from build123d import *

# Parameters (mm, degrees)
BOSS_EXTRUDE1_DEPTH = 30.3
SKETCH2_R           = 2.5527
CUT_EXTRUDE1_DEPTH  = 62.816745304
CUT_EXTRUDE2_DEPTH  = 62.816745304


with BuildPart() as part:
    # Sketch1 → Boss-Extrude1 (new body)
    with BuildSketch(Plane(origin=(0, 0, 0), x_dir=(1, 0, 0), z_dir=(0, 1, 0))):
        Polygon((0, 0), (38.1, 0), (38.1, -18), (18, -18), (18, -38.1), (0, -38.1), align=None)
    extrude(amount=BOSS_EXTRUDE1_DEPTH)

    # Sketch2 → Cut-Extrude1 (cut, through all)
    with BuildSketch(Plane(origin=(0, 30.3, 0), x_dir=(1, 0, 0), z_dir=(0, 1, 0))):
        with Locations(Location((6.35, -6.35, 0), (0, 0, 270))):
            Circle(SKETCH2_R)
        with Locations(Location((19.05, -6.35, 0), (0, 0, 270))):
            Circle(SKETCH2_R)
        with Locations(Location((31.75, -6.35, 0), (0, 0, 270))):
            Circle(SKETCH2_R)
        with Locations(Location((6.35, -19.05, 0), (0, 0, 270))):
            Circle(SKETCH2_R)
        with Locations(Location((6.35, -31.75, 0), (0, 0, 270))):
            Circle(SKETCH2_R)
    extrude(amount=-CUT_EXTRUDE1_DEPTH, mode=Mode.SUBTRACT)

    # Sketch3 → Cut-Extrude2 (cut, through all)
    with BuildSketch(Plane(origin=(0, 30.3, 0), x_dir=(1, 0, 0), z_dir=(0, 1, 0))):
        with BuildLine():
            Line((0, -6.35), (-3.023343313, -6.35))
            Line((-3.023343313, -6.35), (-3.023343313, 2.931868043))
            Line((-3.023343313, 2.931868043), (6.35, 2.931868043))
            Line((6.35, 2.931868043), (6.35, 0))
            ThreePointArc((6.35, 0), (1.859871939, -1.859871939), (0, -6.35))
        make_face()
    extrude(amount=-CUT_EXTRUDE2_DEPTH, mode=Mode.SUBTRACT)


solid = part.part
The listing builds one solid part. Answer for the finished solid, in the listing's coordinates (mm). A direction names the side the tool comes from. Give positions to 0.01 mm unless a question says otherwise; leave off trailing zeros. Loops run counter-clockwise (first coordinate to the right, second up) from the corner with the lowest first, then second, coordinate; pieces in that order, holes last. Notation, with made-up numbers: (-18.5, -21.75) - (-13.5, -21.75) arc R26 cw to (-13.5, 17.25) - close; hole circle Ø8 at (-35.75, -28.5). An arc over 180 degrees is marked (long way). Write each question's results on one line, items separated by ' | '.
1. Find section D-D, the plane x = 5. Write down the section's boundary in (y, z), then the cut area to 3 significant figures.
Resolved:
outline: (0, 0.15) - (30.3, 0.15) - (30.3, 4.18) - (0, 4.18) - close; (0, 8.52) - (30.3, 8.52) - (30.3, 16.88) - (0, 16.88) - close; (0, 21.22) - (30.3, 21.22) - (30.3, 29.58) - (0, 29.58) - close; (0, 33.92) - (30.3, 33.92) - (30.3, 38.1) - (0, 38.1) - close | area: 756 mm^2
2. Find section C-C, the plane x = 31.75. Write down the section's boundary in (y, z), then the cut area to 3 significant figures.
Resolved:
outline: (0, 0) - (30.3, 0) - (30.3, 3.8) - (0, 3.8) - close; (0, 8.9) - (30.3, 8.9) - (30.3, 18) - (0, 18) - close | area: 391 mm^2
3. For a pull along Z with two mould halves and no side action, classify faces 3 (the face through (9, 15, 38.1)), 4 (the face through (38.1, 15, 9)), 5 (the face through (4.085, 15.362, 7.528)) as +Z half, -Z half, draft (parallel to the pull), parting line (faces both ways), or undercut.
Resolved:
face 3: +Z half | face 4: draft | face 5: undercut
4. Find section A-A, the plane y = 26. Write down the section's boundary in (x, z).
Resolved:
outline: (0, 6.35) arc R6.35 ccw to (6.35, 0) - (38.1, 0) - (38.1, 18) - (18, 18) - (18, 38.1) - (0, 38.1) - close; hole circle Ø5.11 at (6.35, 6.35); hole circle Ø5.11 at (6.35, 19.05); hole circle Ø5.11 at (6.35, 31.75); hole circle Ø5.11 at (19.05, 6.35); hole circle Ø5.11 at (31.75, 6.35)
5. Flat-ended cylindrical pins translate along their axes: P1, Ø5, axis at y = 19.5, z = 18.5, coming from the -X side; P2, Ø1, axis at x = 33, y = 16, coming from the +Z side; P3, Ø16, axis at y = 10, z = 32, coming from the +X side. Find the tip coordinate at first contact, or state that the pin passes through.
Resolved:
P1: stops at x = 0 | P2: stops at z = 18 | P3: stops at x = 18
6. Find section B-B, the plane z = 31.75. Write down the section's boundary in (x, y).
Resolved:
outline: (0, 0) - (3.8, 0) - (3.8, 30.3) - (0, 30.3) - close; (8.9, 0) - (18, 0) - (18, 30.3) - (8.9, 30.3) - close
7. Which of the six approach directions +Z, -Z, +X, -X, +Y, -Y give full straight-line access (tool end or side, diameter ignored) to faces 1 (the face through (1.91, 15.36, 1.81)), 2 (the face through (28, 15, 18))?
Resolved:
face 1: -Z, -X, +Y, -Y | face 2: +Z, +X, +Y, -Y
8. Consider probe 1 along X at (y, z) = (21, 6.35); probe 2 along X at (y, z) = (11, 19.05); probe 3 along X at (y, z) = (4.5, 8). Determine where each line is inside the solid, lowest interval first. Write a range as from..to.
Resolved:
probe 1: x = 0..3.8, 8.9..16.5, 21.6..29.2, 34.3..38.1 | probe 2: x = 0..3.8, 8.9..18 | probe 3: x = 0..4.4, 8.3..17.1, 21..29.8, 33.7..38.1
